Verification items for the finished model (mm, model axes). A direction names the side the tool comes from. Round coordinates to 2 decimals unless told otherwise and drop trailing zeros. Write each loop counter-clockwise with the first axis right and the second up, starting at its lowest first coordinate (ties: lowest second). Pieces come first, ordered by that corner, then holes. Notation, with made-up numbers: M 76.25,45.5 L 101.25,45.5 A26 ccw 101.25,62.5 Z; hole C 15.25,35 d5. An arc over 180 degrees is marked long. One line per item, written item: value. Start each with the question number.
Item 1: Section check A-A, the plane z = 4.5. Record the cut outline in (x, y) (3 decimals), then the cut area to 3 significant figures.
Item 2: Section check D-D, the plane y = 3.5. Record the cut outline in (x, z), then the cut area to 3 significant figures.
Item 3: Tool access check on faces 1 (the face through (11.893, -8.295, 3.451)), 2 (the face through (-23.31, -19.07, 3.45)), 3 (the face through (-16, 2, 3)). Record the directions out of +Z, -Z, +X, -X, +Y, -Y that give a thin tool (end or side, any length) a straight path to the whole face; none if there is none.
Item 4: Section check C-C, the plane x = -39.5. Record the cut outline in (y, z).
Item 5: Gauge pin test, flat ends, axial feed: pin 1 (3 mm diameter, centred on x = 33.5, z = 4.5, fed in from -Y); pin 2 (4 mm diameter, centred on x = -26, y = 5, fed in from -Z); pin 3 (1 mm diameter, centred on y = 1.5, z = 3.5, fed in from +X); pin 4 (3 mm diameter, centred on x = 9.5, z = 3, fed in from -Y). Record the tip position at first contact, or that the pin passes through.
Item 6: Thickness scan on probe 1 along Y at (x, z) = (0, 2) (3 decimals); probe 2 along Y at (x, z) = (-27.5, 6.75); probe 3 along X at (y, z) = (-1.5, 1.5). Record the ranges inside material, lowest first. Write a range as from..to.
Item 7: Section check B-B, the plane x = 21.5. Record the cut outline in (y, z), then the cut area to 3 significant figures.
Item 8: Draft check along Y on faces 4 (the face through (8.68, 19.51, 3.45)), 5 (the face through (-0.21, -11.33, 0)), 6 (the face through (16, -2, 3)). Enter one of: +Y half, -Y half, draft (parallel to the pull), parting line (faces both ways), or undercut.
from build123d import *

# Parameters (mm, degrees)
F0_R     = 11.175
F1_DEPTH = 7


# Not quite as in the source:
# - a feature names something its author has since deleted; it is built from what else it names


with BuildPart() as f1:
    # F0 (on Top) → F1 (new body)
    with BuildSketch(Plane.XY):
        with BuildLine():
            ThreePointArc((14.3614066163, -2), (14.465310158, -1.0023981402), (14.5, 0))
            ThreePointArc((14.5, 0), (14.465310158, 1.0023981402), (14.3614066163, 2))
            ThreePointArc((14.3614066163, 2), (11.9468943762, 8.2171597748), (7.0047576617, 12.6958012784))
            ThreePointArc((7.0047576617, 12.6958012784), (3.6166891948, 14.0417078473), (0, 14.5))
            ThreePointArc((0, 14.5), (-3.6166891948, 14.0417078473), (-7.0047576617, 12.6958012784))
            ThreePointArc((-7.0047576617, 12.6958012784), (-11.9468943762, 8.2171597748), (-14.3614066163, 2))
            ThreePointArc((-14.3614066163, 2), (-14.5, 0), (-14.3614066163, -2))
            ThreePointArc((-14.3614066163, -2), (-11.9468943762, -8.2171597748), (-7.0047576617, -12.6958012784))
            ThreePointArc((-7.0047576617, -12.6958012784), (-3.6166891948, -14.0417078473), (0, -14.5))
            ThreePointArc((0, -14.5), (3.6166891948, -14.0417078473), (7.0047576617, -12.6958012784))
            ThreePointArc((7.0047576617, -12.6958012784), (11.9468943762, -8.2171597748), (14.3614066163, -2))
        make_face()
        Circle(F0_R, mode=Mode.SUBTRACT)
        with BuildLine():
            ThreePointArc((14.3614066163, 2), (14.465310158, 1.0023981402), (14.5, 0))
            ThreePointArc((14.5, 0), (14.465310158, -1.0023981402), (14.3614066163, -2))
            Line((14.3614066163, -2), (16.8614066163, -2))
            ThreePointArc((16.8614066163, -2), (16.7228132327, 0), (16.8614066163, 2))
            Line((16.8614066163, 2), (14.3614066163, 2))
        make_face()
        with BuildLine():
            ThreePointArc((0, 14.5), (3.6166891948, 14.0417078473), (7.0047576617, 12.6958012784))
            Line((7.0047576617, 12.6958012784), (1.9398969045, 15.62))
            Line((1.9398969045, 15.62), (0, 14.5))
        make_face()
        with BuildLine():
            ThreePointArc((31.2228132327, 14.5), (21.7030968504, 10.9373214271), (16.8614066163, 2))
            ThreePointArc((16.8614066163, 2), (16.7228132327, 0), (16.8614066163, -2))
            ThreePointArc((16.8614066163, -2), (21.7030968504, -10.9373214271), (31.2228132327, -14.5))
            ThreePointArc((31.2228132327, -14.5), (34.8395024275, -14.0417078473), (38.2275708944, -12.6958012784))
            ThreePointArc((38.2275708944, -12.6958012784), (43.709185526, -7.3716013832), (45.7228132327, 0))
            ThreePointArc((45.7228132327, 0), (43.709185526, 7.3716013832), (38.2275708944, 12.6958012784))
            ThreePointArc((38.2275708944, 12.6958012784), (34.8395024275, 14.0417078473), (31.2228132327, 14.5))
        make_face()
        with Locations((31.2228132327, 0)):
            Circle(F0_R, mode=Mode.SUBTRACT)
        with BuildLine():
            Line((1.9398969045, -15.62), (7.0047576617, -12.6958012784))
            ThreePointArc((7.0047576617, -12.6958012784), (3.6166891948, -14.0417078473), (0, -14.5))
            Line((0, -14.5), (1.9398969045, -15.62))
        make_face()
        Polygon((-1.9398969045, 15.62), (0, 14.5), (1.9398969045, 15.62), (0, 16.74), align=None)
        with BuildLine():
            ThreePointArc((-7.0047576617, 12.6958012784), (-3.6166891948, 14.0417078473), (0, 14.5))
            Line((0, 14.5), (-1.9398969045, 15.62))
            Line((-1.9398969045, 15.62), (-7.0047576617, 12.6958012784))
        make_face()
        Polygon((0, 16.74), (1.9398969045, 15.62), (15.6114066163, 23.5132498124), (15.6114066163, 25.7532498124), align=None)
        with BuildLine():
            Line((15.6114066163, 23.5132498124), (31.2228132327, 14.5))
            ThreePointArc((31.2228132327, 14.5), (34.8395024275, 14.0417078473), (38.2275708944, 12.6958012784))
            Line((38.2275708944, 12.6958012784), (15.6114066163, 25.7532498124))
            Line((15.6114066163, 25.7532498124), (15.6114066163, 23.5132498124))
        make_face()
        with BuildLine():
            Line((-1.9398969045, -15.62), (0, -14.5))
            ThreePointArc((0, -14.5), (-3.6166891948, -14.0417078473), (-7.0047576617, -12.6958012784))
            Line((-7.0047576617, -12.6958012784), (-1.9398969045, -15.62))
        make_face()
        Polygon((1.9398969045, -15.62), (0, -14.5), (-1.9398969045, -15.62), (0, -16.74), align=None)
        Polygon((0, -16.74), (-1.9398969045, -15.62), (-15.6114066163, -23.5132498124), (-15.6114066163, -25.7532498124), align=None)
        with BuildLine():
            ThreePointArc((-14.3614066163, -2), (-14.5, 0), (-14.3614066163, 2))
            Line((-14.3614066163, 2), (-16.8614066163, 2))
            ThreePointArc((-16.8614066163, 2), (-16.7575030746, 1.0023981402), (-16.7228132327, 0))
            ThreePointArc((-16.7228132327, 0), (-16.7575030746, -1.0023981402), (-16.8614066163, -2))
            Line((-16.8614066163, -2), (-14.3614066163, -2))
        make_face()
        with BuildLine():
            Line((-15.6114066163, -25.7532498124), (-15.6114066163, -23.5132498124))
            Line((-15.6114066163, -23.5132498124), (-31.2228132327, -14.5))
            ThreePointArc((-31.2228132327, -14.5), (-34.8395024275, -14.0417078473), (-38.2275708944, -12.6958012784))
            Line((-38.2275708944, -12.6958012784), (-15.6114066163, -25.7532498124))
        make_face()
        with BuildLine():
            ThreePointArc((-16.7228132327, 0), (-16.7575030746, 1.0023981402), (-16.8614066163, 2))
            ThreePointArc((-16.8614066163, 2), (-21.7030968504, 10.9373214271), (-31.2228132327, 14.5))
            ThreePointArc((-31.2228132327, 14.5), (-34.8395024275, 14.0417078473), (-38.2275708944, 12.6958012784))
            ThreePointArc((-38.2275708944, 12.6958012784), (-45.7228132327, 0), (-38.2275708944, -12.6958012784))
            ThreePointArc((-38.2275708944, -12.6958012784), (-34.8395024275, -14.0417078473), (-31.2228132327, -14.5))
            ThreePointArc((-31.2228132327, -14.5), (-21.7030968504, -10.9373214271), (-16.8614066163, -2))
            ThreePointArc((-16.8614066163, -2), (-16.7575030746, -1.0023981402), (-16.7228132327, 0))
        make_face()
        with Locations((-31.2228132327, 0)):
            Circle(F0_R, mode=Mode.SUBTRACT)
    extrude(amount=F1_DEPTH)


solid = f1.part
Response values:
1. outline: M -38.228,-12.696 L -15.611,-25.753 L 7.005,-12.696 A14.5 ccw 14.361,-2 L 16.861,-2 A14.5 ccw long 38.228,12.696 L 15.611,25.753 L -7.005,12.696 A14.5 ccw -14.361,2 L -16.861,2 A14.5 ccw long Z; hole C -31.223,0 d22.35; hole M -31.223,-14.5 L -15.611,-23.513 L -1.94,-15.62 L -7.005,-12.696 A14.5 cw -14.361,-2 L -16.861,-2 A14.5 cw Z; hole C 0,0 d22.35; hole M 1.94,15.62 L 7.005,12.696 A14.5 cw 14.361,2 L 16.861,2 A14.5 cw 31.223,14.5 L 15.611,23.513 Z; hole C 31.223,0 d22.35
1. area: 992 mm2
2. outline: M -45.29,0 L -41.84,0 L -41.84,7 L -45.29,7 Z; M -20.61,0 L -17.15,0 L -17.15,7 L -20.61,7 Z; M -14.07,0 L -10.61,0 L -10.61,7 L -14.07,7 Z; M 10.61,0 L 14.07,0 L 14.07,7 L 10.61,7 Z; M 17.15,0 L 20.61,0 L 20.61,7 L 17.15,7 Z; M 41.84,0 L 45.29,0 L 45.29,7 L 41.84,7 Z
2. area: 145 mm2
3. face 1: +Z, -Z, -Y
3. face 2: +Z, -Z
3. face 3: +Z, -Z, +Y
4. outline: M -11.91,0 L -7.51,0 L -7.51,7 L -11.91,7 Z; M 7.51,0 L 11.91,0 L 11.91,7 L 7.51,7 Z
5. pin 1: stops at y = -14.48
5. pin 2: passes through
5. pin 3: stops at x = 45.69
5. pin 4: stops at y = -12.09
6. probe 1: y = -16.74..-11.175, 11.175..16.74
6. probe 2: y = -18.89..-16.65, -14.01..-10.54, 10.54..14.01
6. probe 3: x = -45.65..-42.3, -20.15..-11.07, 11.07..20.15, 42.3..45.65
7. outline: M -10.76,0 L -5.51,0 L -5.51,7 L -10.76,7 Z; M 5.51,0 L 10.76,0 L 10.76,7 L 5.51,7 Z; M 20.11,0 L 22.35,0 L 22.35,7 L 20.11,7 Z
7. area: 89.2 mm2
8. face 4: undercut
8. face 5: draft
8. face 6: -Y half
